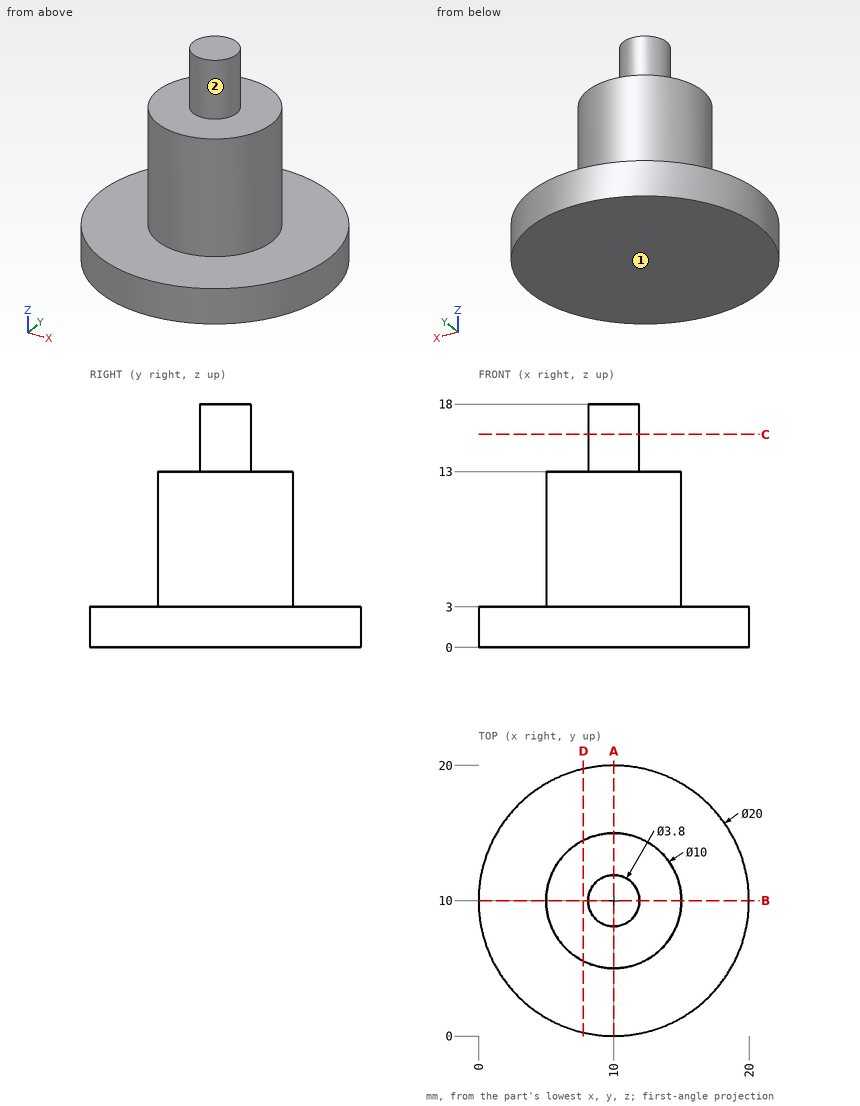
Input: dimensioned drawing with shaded views. Units: mm. Origin: part minimum x, y, z. A direction names the side the tool comes from. Round coordinates to 2 decimals unless told otherwise and drop trailing zeros. Loops run counter-clockwise (first coordinate to the right, second up) from the corner with the lowest first, then second, coordinate; pieces in that order, holes last. Notation, with made-up numbers: (5, 6) -> (25, 6) arc R29 cw to (25, 42) -> close; hole circle Ø8 at (42, 44.25). An arc over 180 degrees is marked (long way). One line per item, written item: value.
(1) Section D-D (x = 7.75). Return the cut outline in (y, z).
Geometry check:
outline: (0.26, 0) -> (19.74, 0) -> (19.74, 3) -> (14.47, 3) -> (14.47, 13) -> (5.53, 13) -> (5.53, 3) -> (0.26, 3) -> close
(2) Section A-A (x = 10). Return the cut outline in (y, z), plus the area to 3 significant figures.
Geometry check:
outline: (0, 0) -> (20, 0) -> (20, 3) -> (15, 3) -> (15, 13) -> (11.9, 13) -> (11.9, 18) -> (8.1, 18) -> (8.1, 13) -> (5, 13) -> (5, 3) -> (0, 3) -> close
area: 179 mm2
(3) Set-up query: the marked faces 1 and 2. Return all of +Z, -Z, +X, -X, +Y, -Y with unobstructed straight access to the full face (end or side cutting, diameter ignored); none if empty.
Geometry check:
face 1: -Z, +X, -X, +Y, -Y
face 2: +Z
(4) Material intervals for line 1 (Z direction, x = 10.5, y = 1.5); line 2 (Y direction, x = 10.25, z = 10.75); line 3 (Y direction, x = 15.5, z = 1.25), sorted ascending. Write a range as [from, to].
Geometry check:
line 1: [0, 3]
line 2: [5.01, 14.99]
line 3: [1.65, 18.35]
(5) Pin query (flat end, axial travel): pin 1 (1 mm diameter, centred on y = 6, z = 8, fed in from +X); pin 2 (3 mm diameter, centred on x = 14, y = 11.5, fed in from +Z); pin 3 (3 mm diameter, centred on x = 5, z = 2.5, fed in from -Y); pin 4 (1 mm diameter, centred on y = 16, z = 7.5, fed in from -X). Return the tip coordinate at first contact, or that it passes through.
Geometry check:
pin 1: x = 13.57
pin 2: z = 13
pin 3: y = 0.63
pin 4: through
(6) Section C-C (z = 15.75). Return the cut outline in (x, y).
Geometry check:
outline: circle Ø3.8 at (10, 10)
